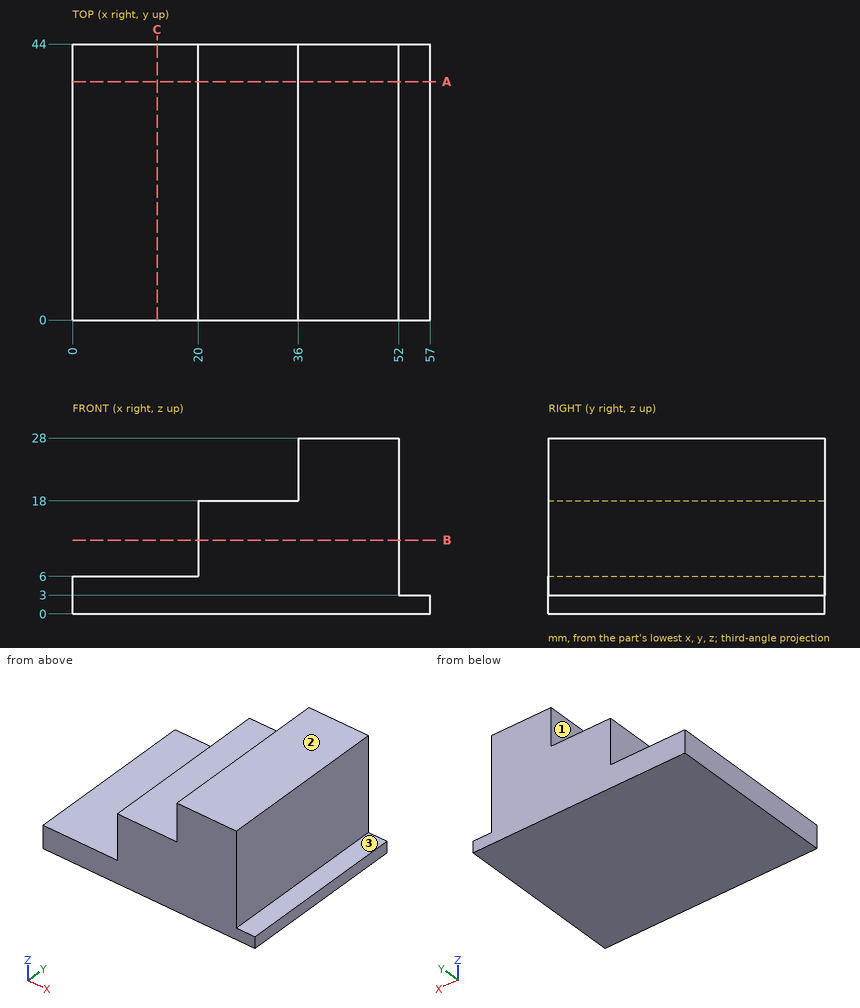
Input: dimensioned drawing with shaded views. Units: mm. Origin: part minimum x, y, z. A direction names the side the tool comes from. Coordinates: 2 decimals unless noted, no trailing zeros. Order: outer loops, then holes, each group sorted by start corner. A loop starts at its lowest first (then second) coordinate and runs counter-clockwise, first axis right, second up. Notation, with made-up numbers: (0.25, 11.25) - (26.25, 11.25) arc R18 ccw to (26.25, 17.25) - close; hole circle Ø5 at (56, 1). An arc over 180 degrees is marked (long way). One line per item, written item: value.
1) Cut plane B-B on z = 11.75. Output: boundary loops of the cut face in (x, y).
Computed values:
outline: (20, 0) - (52, 0) - (52, 44) - (20, 44) - close
2) Contact query for flat-ended pins moving along their axis: pin 1 (10 mm diameter, centred on x = 9.5, y = 24, fed in from +Z); pin 2 (3 mm diameter, centred on x = 21.5, y = 34.5, fed in from +Z); pin 3 (5 mm diameter, centred on y = 15.5, z = 23, fed in from -X); pin 4 (10 mm diameter, centred on x = 7.5, z = 13.5, fed in from -Y). Output: stop coordinate, or through.
Computed values:
pin 1: stops at z = 6
pin 2: stops at z = 18
pin 3: stops at x = 36
pin 4: passes through
3) Reachability of the marked faces 1, 2 and 3 from +Z, -Z, +X, -X, +Y, -Y: full face, straight path, thin tool, end or side. Return the list, or none.
Computed values:
face 1: +Z, -X, +Y, -Y
face 2: +Z, +X, -X, +Y, -Y
face 3: +Z, +X, +Y, -Y
4) Cut plane A-A on y = 38. Output: boundary loops of the cut face in (x, z).
Computed values:
outline: (0, 0) - (57, 0) - (57, 3) - (52, 3) - (52, 28) - (36, 28) - (36, 18) - (20, 18) - (20, 6) - (0, 6) - close
5) Cut plane C-C on x = 13.5. Output: boundary loops of the cut face in (y, z).
Computed values:
outline: (0, 0) - (44, 0) - (44, 6) - (0, 6) - close
6) Ray query, line 1 (X direction, y = 11.5, z = 8.25); line 2 (X direction, y = 13, z = 5.75); line 3 (Z direction, x = 9.5, y = 23). Return the intervals inside material, ascending. Write a range as [from, to].
Computed values:
line 1: x = [20, 52]
line 2: x = [0, 52]
line 3: z = [0, 6]
